Source: CAD feature listing. Evaluate the final solid. Frame: model axes, mm. Face numbers are marked on the shaded views. Coordinates: 2 decimals unless noted, no trailing zeros. Write each loop counter-clockwise with the first axis right and the second up, starting at its lowest first coordinate (ties: lowest second). Pieces come first, ordered by that corner, then holes. Notation, with made-up numbers: (27, 86.5) - (39, 86.5) arc R19 cw to (39, 105.5) - close; hole circle Ø8 at (-28, 25). An arc over 180 degrees is marked (long way). One line per question, with ' | ' between items.
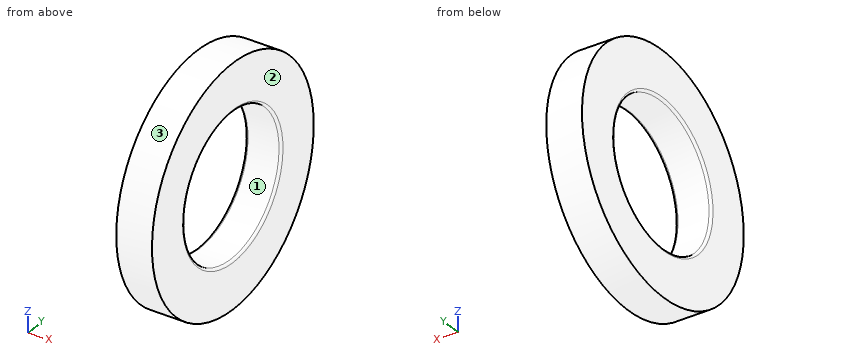
from build123d import *

# Parameters (mm, degrees)
ESBO_O2_R                = 50
RESSALTO_EXTRUS_O1_DEPTH = 15
ESBO_O3_R                = 30
CORTE_EXTRUS_O1_DEPTH    = 73.284161474
FILETE1_R                = 1


with BuildPart() as part:
    # Esboço2 → Ressalto-extrusão1 (new body)
    with BuildSketch(Plane(origin=(0, 0, 0), x_dir=(0, 0, -1), z_dir=(1, 0, 0))):
        Circle(ESBO_O2_R)
    extrude(amount=RESSALTO_EXTRUS_O1_DEPTH)

    # Esboço3 → Corte-extrusão1 (cut, through all)
    with BuildSketch(Plane(origin=(15, 0, 0), x_dir=(0, 0, -1), z_dir=(1, 0, 0))):
        Circle(ESBO_O3_R)
    extrude(amount=-CORTE_EXTRUS_O1_DEPTH, mode=Mode.SUBTRACT)

    # Filete1
    filete1_edges = [part.edges().sort_by_distance(p)[0] for p in [
        (0, 0, 30),
        (15, 0, 30),
    ]]
    fillet(filete1_edges, radius=FILETE1_R)


solid = part.part
Item 1: Mould query, pull axis Z, two halves, no side actions, for the marked faces 1, 2 and 3. Classes: pulls with the +Z half, pulls with the -Z half, needs draft (parallel to the pull), parting line crosses it, or undercut.
Check sheet entries:
face 1: undercut | face 2: needs draft | face 3: parting line crosses it
Item 2: Pin query (flat end, axial travel): pin 1 Ø4 at (x, y) = (13.5, -24) entering from +Z; pin 2 Ø3 at (x, z) = (2.5, 2) entering from -Y; pin 3 Ø1 at (x, y) = (13.5, 18) entering from +Z; pin 4 Ø12 at (y, z) = (13, -36.5) entering from -X. Return the tip coordinate at first contact, or that it passes through.
Check sheet entries:
pin 1: z = 44.9 | pin 2: y = -50 | pin 3: z = 46.84 | pin 4: x = 0
Item 3: Ray query, line 1 along Y through (x, z) = (3.75, 0); line 2 along Z through (x, y) = (5.75, -1); line 3 along Z through (x, y) = (3.25, 18.5). Return the intervals inside material, ascending. Write a range as [from, to].
Check sheet entries:
line 1: [-50, -30], [30, 50] | line 2: [-49.99, -29.98], [29.98, 49.99] | line 3: [-46.45, -23.62], [23.62, 46.45]
Item 4: Cut plane A-A on y = 0. Return loops of the section in (x, z), and give its area (3 significant figures).
Check sheet entries:
outline: (0, -50) - (15, -50) - (15, -31) arc R1 ccw to (14, -30) - (1, -30) arc R1 ccw to (0, -31) - close; (0, 31) arc R1 ccw to (1, 30) - (14, 30) arc R1 ccw to (15, 31) - (15, 50) - (0, 50) - close | area: 599 mm²
Item 5: Cut plane C-C on x = 7.5. Return loops of the section in (y, z).
Check sheet entries:
outline: circle Ø100 at (0, 0); hole circle Ø60 at (0, 0)
Item 6: Cut plane D-D on z = 38. Return loops of the section in (x, y).
Check sheet entries:
outline: (0, -32.5) - (15, -32.5) - (15, 32.5) - (0, 32.5) - close
